```python
from build123d import *

# Parameters (mm, degrees)
F0_R     = 7.95655
F1_DEPTH = 27.94
F2_R     = 7.1755
F3_DEPTH = 76.2
F5_R     = 1.5875
F6_DEPTH = 12.7
F7_SIZE  = 0.508
F8_SIZE2 = 1.4516166425
F8_SIZE  = 0.127


with BuildPart() as f1:
    # F0 (on Top) → F1 (new body)
    with BuildSketch(Plane.XY):
        Circle(F0_R)
    extrude(amount=F1_DEPTH)

    # F2 (on face) → F3 (join)
    with BuildSketch(Plane.XY.offset(27.94)):
        Circle(F2_R)
    extrude(amount=F3_DEPTH)

    # F5 (on face) → F6 (cut, symmetric)
    with BuildSketch(Plane.YZ):
        with Locations((0, 99.06)):
            Circle(F5_R)
    extrude(amount=F6_DEPTH, both=True, mode=Mode.SUBTRACT)

    # F7
    f7_edges = [f1.edges().sort_by_distance(p)[0] for p in [
        (-7.1755, 0, 104.14),
    ]]
    chamfer(f7_edges, length=F7_SIZE)

    # F8
    f8_edges = [f1.edges().sort_by_distance(p)[0] for p in [
        (-7.95655, 0, 0),
    ]]
    f8_side = f1.faces().sort_by_distance((0, 0, 0))[0]
    chamfer(f8_edges, length=F8_SIZE, length2=F8_SIZE2, reference=f8_side)


solid = f1.part
```
The model under review builds one solid part; all positions refer to its coordinate system, in mm. A direction names the side the tool comes from. Round coordinates to 2 decimals unless told otherwise and drop trailing zeros. Loops run counter-clockwise (first coordinate to the right, second up) from the corner with the lowest first, then second, coordinate; pieces in that order, holes last. Notation, with made-up numbers: M 51.5,-15 L 77.5,-15 A16 cw 77.5,5 Z; hole C -7.75,58.5 d2. An arc over 180 degrees is marked long. Put each result on its own line as item: value.
Q1. Consider section D-D, the plane z = 11. Give the boundary of the cut face in (x, y), then the cut area to 3 significant figures.
Result set:
outline: C 0,0 d15.91
area: 199 mm²
Q2. Consider section A-A, the plane y = 0. Give the boundary of the cut face in (x, z).
Result set:
outline: M -7.96,1.45 L -7.83,0 L 7.83,0 L 7.96,1.45 L 7.96,27.94 L 7.18,27.94 L 7.18,97.47 L -7.18,97.47 L -7.18,27.94 L -7.96,27.94 Z; M -7.18,100.65 L 7.18,100.65 L 7.18,103.63 L 6.67,104.14 L -6.67,104.14 L -7.18,103.63 Z
Q3. To check wall thickness, follow L1, parallel to Z at x = 2, y = 0.25; L2, parallel to Z at x = -5, y = 5.5; L3, parallel to Y at x = 1.5, z = 5. State the ranges of each line that lie inside material, in increasing order.
Result set:
L1: z = 0 to 97.49, 100.63 to 104.14
L2: z = 0 to 27.94
L3: y = -7.81 to 7.81
Q4. For pin 1 (2 mm diameter, centred on x = -4, z = 58, fed in from +Y); pin 2 (1 mm diameter, centred on y = -3, z = 90.5, fed in from +X); pin 3 (6 mm diameter, centred on x = -3, z = 69, fed in from +Y), all flat-tipped, find the tip position at first contact; note any pin that passes through.
Result set:
pin 1: stops at y = 6.52
pin 2: stops at x = 6.73
pin 3: stops at y = 7.18
Q5. Mouldability with a two-part tool opening along Z and no side actions: class faces 3 (the flat face through (0, 0, 104.14)), 4 (the flat face through (0, 0, 0)), 5 (the cylindrical face through (0.099, -0.207, 100.634)) as released by +Z, released by -Z, zero draft, split by the parting line, or undercut.
Result set:
face 3: released by +Z
face 4: released by -Z
face 5: undercut
Q6. Consider section B-B, the plane x = 0. Give the boundary of the cut face in (y, z) (1 decimal), then the cut area to 3 significant figures.
Result set:
outline: M -8,1.5 L -7.8,0 L 7.8,0 L 8,1.5 L 8,27.9 L 7.2,27.9 L 7.2,103.6 L 6.7,104.1 L -6.7,104.1 L -7.2,103.6 L -7.2,27.9 L -8,27.9 Z; hole C 0,99.1 d3.2
area: 1,530 mm²
Q7. Consider section C-C, the plane z = 99.06. Give the boundary of the cut face in (x, y).
Result set:
outline: M -7,-1.59 A7.18 ccw 7,-1.59 Z; M -7,1.59 L 7,1.59 A7.18 ccw Z
Q8. Machinability: for faces 1 (the cylindrical face through (-1.72, -7.77, 14.51)), 2 (the flat face through (-1.81, 7.11, 27.94)), which of the approach directions +Z, -Z, +X, -X, +Y, -Y give a long, thin tool a straight path to every point of the face, cutting with its end or side? Answer none if there is none.
Result set:
face 1: +Z, -Z
face 2: +Z
